from build123d import *

# Parameters (mm, degrees)
F0_W     = 273.05
F0_H     = 228.6
F1_DEPTH = 19.05
F3_DEPTH = 19.05
F5_DEPTH = 19.05


with BuildPart() as f1:
    # F0 (on Right) → F1 (new body)
    with BuildSketch(Plane.YZ):
        with Locations((136.525, 114.3)):
            Rectangle(F0_W, F0_H)
    extrude(amount=-F1_DEPTH)

    # F2 (on face) → F3 (cut, through all)
    with BuildSketch(Plane.YZ):
        Polygon((182.0333333333, 139.7), (273.05, 139.7), (273.05, 228.6), (0, 228.6), (0, 0), (91.0166666667, 0), (91.0166666667, 69.85), (182.0333333333, 69.85), align=None)
    extrude(amount=-F3_DEPTH, mode=Mode.SUBTRACT)

    # F4 (on face) → F5 (cut, through all)
    with BuildSketch(Plane.YZ):
        Polygon((110.0666666667, 0), (110.0666666667, 50.8), (201.0833333333, 50.8), (201.0833333333, 120.65), (273.05, 120.65), (273.05, 139.7), (182.0333333333, 139.7), (182.0333333333, 69.85), (91.0166666667, 69.85), (91.0166666667, 0), align=None)
    extrude(amount=-F5_DEPTH, mode=Mode.SUBTRACT)


solid = f1.part
The listing builds one solid part. Answer for the finished solid, in the listing's coordinates (mm). A direction names the side the tool comes from. Give positions to 0.01 mm unless a question says otherwise; leave off trailing zeros. Order: outer loops, then holes, each group sorted by start corner. A loop starts at its lowest first (then second) coordinate and runs counter-clockwise, first axis right, second up. Notation, with made-up numbers: (10, -16) - (35, -16) arc R21 ccw to (35, 13) - close; hole circle Ø6 at (65.25, -40). An arc over 180 degrees is marked (long way). Answer as CSV lines item,"result".
Q1. Straight lines are drawn through the part: L1, parallel to Z at x = -5.25, y = 156.5; L2, parallel to Y at x = -15.75, z = 55. For each, find the intervals that lie inside material, in ascending order.
Answer key:
L1,"z = 0 to 50.8"
L2,"y = 201.08 to 273.05"
Q2. Each of these flat-tipped pins is pushed along its axis until it touches: pin 1 Ø1 at (x, y) = (-13, 177) entering from +Z; pin 2 Ø5.5 at (x, z) = (-7, 100.5) entering from -Y. Where does it stop, or does it pass through?
Answer key:
pin 1,"stops at z = 50.8"
pin 2,"stops at y = 201.08"
Q3. A cutting plane is placed at A-A, the plane y = 196.5. Determine the outline of the cut face in (x, z), and give its area (3 significant figures).
Answer key:
outline,"(-19.05, 0) - (0, 0) - (0, 50.8) - (-19.05, 50.8) - close"
area,"968 mm^2"
Q4. A cutting plane is placed at B-B, the plane x = -5.5. Determine the outline of the cut face in (y, z), and give its area (3 significant figures).
Answer key:
outline,"(110.07, 0) - (273.05, 0) - (273.05, 120.65) - (201.08, 120.65) - (201.08, 50.8) - (110.07, 50.8) - close"
area,"13,300 mm^2"
Q5. A cutting plane is placed at C-C, the plane z = 94.5. Determine the outline of the cut face in (x, y).
Answer key:
outline,"(-19.05, 201.08) - (0, 201.08) - (0, 273.05) - (-19.05, 273.05) - close"
Q6. Which of the six approach directions +Z, -Z, +X, -X, +Y, -Y give full straight-line access (tool end or side, diameter ignored) to faces 1 (the face through (-9, 237, 120.65)), 2 (the face through (-9, 201.083, 85))?
Answer key:
face 1,"+Z, +X, -X, +Y, -Y"
face 2,"+Z, +X, -X, -Y"
